from build123d import *

# Parameters (mm, degrees)
SKETCH_1_W           = 40
SKETCH_1_H           = 97
EXTRUDE_1_DEPTH      = 1
F_4_0MM_1_AT_2_COUNT = 2
F_4_0MM_1_AT_2_PITCH = 15
EXTRUDE_START        = -1
SKETCH_6_2_W         = 186
SKETCH_6_2_H         = 97
EXTRUDE_3_DEPTH      = 3
FILLET_2_R           = 36.5
SKETCH_8_W           = 22
SKETCH_8_H           = 45
CUT_EXTRUDE_2_DEPTH  = 105.929738397


with BuildPart() as part:
    # 草圖1 → 填料-伸長1 (new body)
    with BuildSketch(Plane(origin=(0, 0, 0), x_dir=(1, 0, 0), z_dir=(0, 1, 0))):
        Rectangle(SKETCH_1_W, SKETCH_1_H)
    extrude(amount=EXTRUDE_1_DEPTH)

    # 草圖5 → Ø4.0mm 定位孔1 (revolve, cut)
    with BuildSketch(Plane(origin=(7.5, 1, 0), x_dir=(0, 0, 1), z_dir=(1, 0, 0))):
        Polygon((0, 0), (0, 1), (2, 1), (2, 0.025), (2.025, 0), align=None)
    f_4_0mm_1 = revolve(axis=Axis((7.5, 7.35, 0), (0, -1, 0)), mode=Mode.SUBTRACT)

    # Ø4.0mm 定位孔1 at 2: Ø4.0mm 定位孔1 ×2
    with Locations(*[(-i * F_4_0MM_1_AT_2_PITCH, 0, 0) for i in range(1, F_4_0MM_1_AT_2_COUNT)]):
        add(f_4_0mm_1, mode=Mode.SUBTRACT)

    # 草圖6<2> → 填料-伸長3 (add)
    with BuildSketch(Plane(origin=(0, 1, 0), x_dir=(1, 0, 0), z_dir=(0, 1, 0)).offset(EXTRUDE_START)):
        Rectangle(SKETCH_6_2_W, SKETCH_6_2_H)
    extrude(amount=-EXTRUDE_3_DEPTH)

    # 圓角2
    fillet_2_edges = [part.edges().sort_by_distance(p)[0] for p in [
        (-93, -1.5, -48.5),
        (93, -1.5, -48.5),
    ]]
    fillet(fillet_2_edges, radius=FILLET_2_R)

    # 草圖8 → 除料-伸長2 (cut, through all)
    with BuildSketch(Plane(origin=(0, 0, 0), x_dir=(1, 0, 0), z_dir=(0, 1, 0))):
        with Locations((-82, -26)):
            Rectangle(SKETCH_8_W, SKETCH_8_H)
    extrude(amount=-CUT_EXTRUDE_2_DEPTH, mode=Mode.SUBTRACT)


solid = part.part
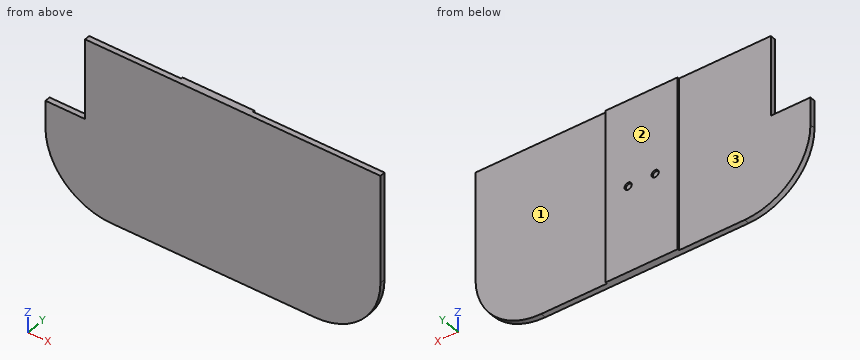
Verification items for the finished model (mm, model axes). Face numbers are marked on the shaded views. A direction names the side the tool comes from. Give positions to 0.01 mm unless a question says otherwise; leave off trailing zeros. Order: outer loops, then holes, each group sorted by start corner. A loop starts at its lowest first (then second) coordinate and runs counter-clockwise, first axis right, second up. Notation, with made-up numbers: M -3,18.25 L 9,18.25 A9 ccw 9,35.25 Z; hole C 61.25,9.25 d9. An arc over 180 degrees is marked long. Answer as a JSON object with one key per item and string values. Group by question number.
1) Cross-section at D-D (z = 21.5). Enter the section's corners in (x, y), then the cut area to 3 significant figures.
2) Scan lines: line 1 along X through (y, z) = (0.5, 0); line 2 along Z through (x, y) = (-7.5, 0.6); line 3 along Y through (x, z) = (68.5, -18.5). Record each from-to range of solid material in increasing order. Write a range as [from, to].
3) Cross-section at A-A (z = 0). Enter the section's corners in (x, y) (3 decimals), then the cut area to 3 significant figures.
4) Depth check by flat-ended pin: pin 1 Ø0.9 at (y, z) = (-1, 30.5) entering from -X; pin 2 Ø8 at (x, z) = (-33.5, -22.5) entering from +Y; pin 3 Ø0.8 at (y, z) = (0.5, 19.5) entering from +X. Enter the tip coordinate at first touch or a pass-through.
5) Cross-section at B-B (y = -2.1). Enter the section's corners in (x, z), then the cut area to 3 significant figures.
6) Access from +Z, -Z, +X, -X, +Y, -Y to the whole of each face (thin tool, end or side, straight path). Record for the marked faces 1, 2 and 3.
7) Cross-section at C-C (x = -52). Enter the section's corners in (y, z).
Result sheet:
{
 "1": {"outline": "M -71,-3 L 93,-3 L 93,0 L 20,0 L 20,1 L -20,1 L -20,0 L -71,0 Z", "area": "532 mm2"},
 "2": {"line 1": "x = [-20, -9.5], [-5.5, 5.5], [9.5, 20]", "line 2": "z = [-48.5, -2], [2, 48.5]", "line 3": "y = [-3, 0]"},
 "3": {"outline": "M -93,-3 L 93,-3 L 93,0 L 20,0 L 20,1 L 9.525,1 L 9.5,0.975 L 9.5,0 L 5.5,0 L 5.5,0.975 L 5.475,1 L -5.475,1 L -5.5,0.975 L -5.5,0 L -9.5,0 L -9.5,0.975 L -9.525,1 L -20,1 L -20,0 L -93,0 Z", "area": "590 mm2"},
 "4": {"pin 1": "stops at x = -71", "pin 2": "stops at y = 0", "pin 3": "stops at x = 20"},
 "5": {"outline": "M -93,-12 A36.5 ccw -56.5,-48.5 L 56.5,-48.5 A36.5 ccw 93,-12 L 93,48.5 L -71,48.5 L -71,3.5 L -93,3.5 Z", "area": "16,500 mm2"},
 "6": {"face 1": "+Z, -Z, +X, +Y", "face 2": "+Z, -Z, +X, -X, +Y", "face 3": "+Z, -Z, -X, +Y"},
 "7": {"outline": "M -3,-48.5 L 0,-48.5 L 0,48.5 L -3,48.5 Z"}
}
